Source: CAD feature listing. Evaluate the final solid. Frame: model axes, mm. Face numbers are marked on the shaded views. Coordinates: 2 decimals unless noted, no trailing zeros. Loops run counter-clockwise (first coordinate to the right, second up) from the corner with the lowest first, then second, coordinate; pieces in that order, holes last.
Item 1: Section query A-A, the plane y = 6. Return the cut outline in (x, z).
Item 2: Section query C-C, the plane x = 10.5. Return the cut outline in (y, z), then the cut area to 3 significant figures.
Item 3: Pin query (flat end, axial travel): pin 1 Ø1 at (x, z) = (3.5, 1.5) entering from -Y; pin 2 Ø2.5 at (x, z) = (-1.5, 1.5) entering from -Y; pin 3 Ø6 at (y, z) = (7, 5.5) entering from +X. Return the tip coordinate at first contact, or that it passes through.
Item 4: Line query: probe 1 along Z at (x, y) = (0, 1.5); probe 2 along Z at (x, y) = (0, 4.75); probe 3 along X at (y, z) = (3.25, 2.5). Output: solid intervals per line, ascending.
Item 5: Section query B-B, the plane z = 0. Return the cut outline in (x, y).
Item 6: Pull-direction query (Z, two-part tool) for the marked faces 1, 2, 3 and 4; classes: +Z half, -Z half, draft (parallel to the pull), parting line (faces both ways), or undercut.
Item 7: Section query D-D, the plane x = 0. Return the cut outline in (y, z), then the cut area to 3 significant figures.
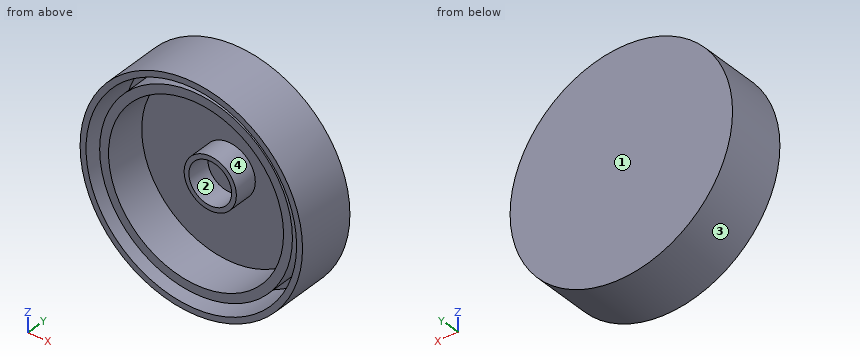
```python
from build123d import *

# Parameters (mm, degrees)
SKETCH002_R      = 18.75
PAD001_DEPTH     = 2
SKETCH003_R      = 4.4
SKETCH003_R_2    = 3.6
PAD002_DEPTH     = 4
SKETCH003001_R   = 16.25
SKETCH003001_R_2 = 14.75
PAD003_DEPTH     = 7
SKETCH003002_R   = 18.75
SKETCH003002_R_2 = 17.75
PAD004_DEPTH     = 8


with BuildPart() as toppad:
    # Sketch002 → Pad001 (new body)
    with BuildSketch(Plane.XZ.offset(-7.8)):
        Circle(SKETCH002_R)
    extrude(amount=-PAD001_DEPTH)


with BuildPart() as centershaft:
    # Sketch003 → Pad002 (new body)
    with BuildSketch(Plane.XZ.offset(-7.8)):
        Circle(SKETCH003_R)
        Circle(SKETCH003_R_2, mode=Mode.SUBTRACT)
    extrude(amount=PAD002_DEPTH)


with BuildPart() as topguidering001:
    # Sketch003001 → Pad003 (new body)
    with BuildSketch(Plane.XZ.offset(-7.8)):
        Circle(SKETCH003001_R)
        Circle(SKETCH003001_R_2, mode=Mode.SUBTRACT)
    extrude(amount=PAD003_DEPTH)


with BuildPart() as topfusion:
    # Sketch003002 → Pad004 (new body)
    with BuildSketch(Plane.XZ.offset(-7.8)):
        Circle(SKETCH003002_R)
        Circle(SKETCH003002_R_2, mode=Mode.SUBTRACT)
    extrude(amount=PAD004_DEPTH)

    # Fusion001: union TopPad, CenterShaft, TopGuideRing001
    add(toppad.part)
    add(centershaft.part)
    add(topguidering001.part)


solid = topfusion.part
```
Verdict:
1. outline: circle Ø37.5 at (0, 0); circle Ø32.5 at (0, 0); circle Ø8.8 at (0, 0); hole circle Ø35.5 at (0, 0); hole circle Ø29.5 at (0, 0); hole circle Ø7.2 at (0, 0)
2. outline: (-0.2, -15.53) - (9.8, -15.53) - (9.8, 15.53) - (-0.2, 15.53) - (-0.2, 14.31) - (7.8, 14.31) - (7.8, 12.4) - (0.8, 12.4) - (0.8, 10.36) - (7.8, 10.36) - (7.8, -10.36) - (0.8, -10.36) - (0.8, -12.4) - (7.8, -12.4) - (7.8, -14.31) - (-0.2, -14.31) - close
2. area: 110 mm2
3. pin 1: stops at y = 3.8
3. pin 2: stops at y = 7.8
3. pin 3: stops at x = 18.58
4. probe 1: z = -18.75 to -17.75, -16.25 to -14.75, 14.75 to 16.25, 17.75 to 18.75
4. probe 2: z = -18.75 to -17.75, -16.25 to -14.75, -4.4 to -3.6, 3.6 to 4.4, 14.75 to 16.25, 17.75 to 18.75
4. probe 3: x = -18.58 to -17.57, -16.06 to -14.54, 14.54 to 16.06, 17.57 to 18.58
5. outline: (-18.75, -0.2) - (-17.75, -0.2) - (-17.75, 7.8) - (-16.25, 7.8) - (-16.25, 0.8) - (-14.75, 0.8) - (-14.75, 7.8) - (-4.4, 7.8) - (-4.4, 3.8) - (-3.6, 3.8) - (-3.6, 7.8) - (3.6, 7.8) - (3.6, 3.8) - (4.4, 3.8) - (4.4, 7.8) - (14.75, 7.8) - (14.75, 0.8) - (16.25, 0.8) - (16.25, 7.8) - (17.75, 7.8) - (17.75, -0.2) - (18.75, -0.2) - (18.75, 9.8) - (-18.75, 9.8) - close
6. face 1: draft
6. face 2: undercut
6. face 3: parting line
6. face 4: undercut
7. outline: (-0.2, -18.75) - (9.8, -18.75) - (9.8, 18.75) - (-0.2, 18.75) - (-0.2, 17.75) - (7.8, 17.75) - (7.8, 16.25) - (0.8, 16.25) - (0.8, 14.75) - (7.8, 14.75) - (7.8, 4.4) - (3.8, 4.4) - (3.8, 3.6) - (7.8, 3.6) - (7.8, -3.6) - (3.8, -3.6) - (3.8, -4.4) - (7.8, -4.4) - (7.8, -14.75) - (0.8, -14.75) - (0.8, -16.25) - (7.8, -16.25) - (7.8, -17.75) - (-0.2, -17.75) - close
7. area: 118 mm2
